Can you work these out from the model? Positions are in its coordinate system, mm. Face numbers are marked on the shaded views. Coordinates: 2 decimals unless noted, no trailing zeros. Loops run counter-clockwise (first coordinate to the right, second up) from the corner with the lowest first, then second, coordinate; pieces in that order, holes last.
```python
from build123d import *

# Parameters (mm, degrees)
CUT_EXTRUDE_316_DEPTH = 1.5


with BuildPart() as part:
    # Sketch 184 → Revolve 217 (revolve)
    with BuildSketch(Plane.XY, mode=Mode.PRIVATE) as revolve_217_sk:
        Polygon((0, 0), (4, 0), (2, 2), (2, 11.7), (1.7, 12), (0, 12), align=None)
    revolve(revolve_217_sk.sketch.rotate(Axis((0, -2, 0), (0, 1, 0)), 90), axis=Axis((0, -2, 0), (0, 1, 0)))

    # Sketch 268 → Cut-Extrude 316 (cut)
    with BuildSketch(Plane.XZ):
        Polygon((1.443375673, 0), (0.721687836, 1.25), (-0.721687836, 1.25), (-1.443375673, 0), (-0.721687836, -1.25), (0.721687836, -1.25), align=None)
    extrude(amount=-CUT_EXTRUDE_316_DEPTH, mode=Mode.SUBTRACT)


solid = part.part
```
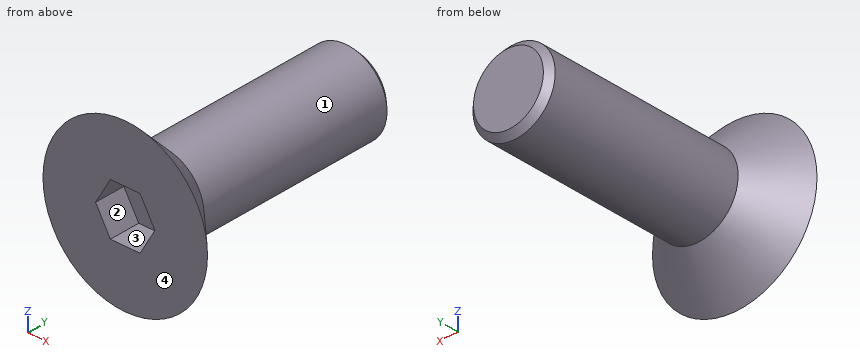
(1) I want a section at C-C on y = 5. Write out the boundary of the cut face in (x, z), then the cut area to 3 significant figures.
Check values:
outline: circle Ø4 at (0, 0)
area: 12.6 mm2
(2) If I drill on probe 1 along Y at (x, z) = (-0.75, -0.25); probe 2 along Z at (x, y) = (-0.5, 8.5); probe 3 along Z at (x, y) = (1.75, 7.75), over which ranges is the centre line in solid material (lowest first)?
Check values:
probe 1: y = 1.5 to 12
probe 2: z = -1.94 to 1.94
probe 3: z = -0.97 to 0.97
(3) I want a section at A-A on y = 1.25. Write out the boundary of the cut face in (x, z).
Check values:
outline: circle Ø5.5 at (0, 0); hole (-1.44, 0) - (-0.72, -1.25) - (0.72, -1.25) - (1.44, 0) - (0.72, 1.25) - (-0.72, 1.25) - close
(4) I'm going to push flat-ended pins straight in: pin 1 (1.2 mm diameter, centred on x = 0, y = 1, fed in from +Z); pin 2 (4 mm diameter, centred on x = 1, z = 0.5, fed in from -Y); pin 3 (4 mm diameter, centred on x = 2, y = 8, fed in from +Z); pin 4 (1.5 mm diameter, centred on y = 6.5, z = -1.5, fed in from +X). Where does each tip first touch, or does it pass through?
Check values:
pin 1: stops at z = 3.6
pin 2: stops at y = 0
pin 3: stops at z = 2
pin 4: stops at x = 1.85
(5) I want a section at B-B on x = 0. Write out the boundary of the cut face in (y, z).
Check values:
outline: (0, -4) - (2, -2) - (11.7, -2) - (12, -1.7) - (12, 1.7) - (11.7, 2) - (2, 2) - (0, 4) - (0, 1.25) - (1.5, 1.25) - (1.5, -1.25) - (0, -1.25) - close
(6) If we mould it in two halves opening along X, with no side actions, what happens to the marked faces 1, 2, 3 and 4? For each: released by +X, released by -X, zero draft, split by the parting line, or undercut.
Check values:
face 1: split by the parting line
face 2: undercut
face 3: undercut
face 4: zero draft
